```python
from build123d import *

# Parameters (mm, degrees)
BASE_PLATE_AND_PORTS_2_R   = 0.35
BASE_PLATE_AND_PORTS_2_R_2 = 1.075
BASE_PLATE_AND_PORTS_DEPTH = 1.5
BOSS_EXTRUDE1_DEPTH        = 15
RESERVOIRS_3_W             = 0.5
RESERVOIRS_3_H             = 12
BOSS_EXTRUDE2_DEPTH        = 13


with BuildPart() as part:
    # Base-plate and ports 2 → Base plate and ports (new, symmetric)
    with BuildSketch(Plane(origin=(0, 0, 0), x_dir=(1, 0, 0), z_dir=(0, 1, 0))):
        with BuildLine():
            Line((-16, -7), (-16, 7))
            ThreePointArc((-16, 7), (-15.560660172, 8.060660172), (-14.5, 8.5))
            Line((-14.5, 8.5), (-3.175, 8.5))
            ThreePointArc((-3.175, 8.5), (-2.379504871, 8.829504871), (-2.05, 9.625))
            ThreePointArc((-2.05, 9.625), (0, 11.675), (2.05, 9.625))
            ThreePointArc((2.05, 9.625), (2.379504871, 8.829504871), (3.175, 8.5))
            Line((3.175, 8.5), (14.5, 8.5))
            ThreePointArc((14.5, 8.5), (15.560660172, 8.060660172), (16, 7))
            Line((16, 7), (16, -7))
            ThreePointArc((16, -7), (15.560660172, -8.060660172), (14.5, -8.5))
            Line((14.5, -8.5), (12.175, -8.5))
            ThreePointArc((12.175, -8.5), (11.379504871, -8.829504871), (11.05, -9.625))
            ThreePointArc((11.05, -9.625), (9, -11.675), (6.95, -9.625))
            ThreePointArc((6.95, -9.625), (6.620495129, -8.829504871), (5.825, -8.5))
            Line((5.825, -8.5), (-5.825, -8.5))
            ThreePointArc((-5.825, -8.5), (-6.620495129, -8.829504871), (-6.95, -9.625))
            ThreePointArc((-6.95, -9.625), (-9, -11.675), (-11.05, -9.625))
            ThreePointArc((-11.05, -9.625), (-11.379504871, -8.829504871), (-12.175, -8.5))
            Line((-12.175, -8.5), (-14.5, -8.5))
            ThreePointArc((-14.5, -8.5), (-15.560660172, -8.060660172), (-16, -7))
        make_face()
        with Locations(Location((-10.5, 3, 0), (0, 0, 270))):
            Circle(BASE_PLATE_AND_PORTS_2_R, mode=Mode.SUBTRACT)
        with Locations(Location((0, 3, 0), (0, 0, 270))):
            Circle(BASE_PLATE_AND_PORTS_2_R, mode=Mode.SUBTRACT)
        with Locations(Location((10.5, 3, 0), (0, 0, 270))):
            Circle(BASE_PLATE_AND_PORTS_2_R, mode=Mode.SUBTRACT)
        with Locations(Location((0, -3, 0), (0, 0, 270))):
            Circle(BASE_PLATE_AND_PORTS_2_R, mode=Mode.SUBTRACT)
        with Locations(Location((10.5, -3, 0), (0, 0, 270))):
            Circle(BASE_PLATE_AND_PORTS_2_R, mode=Mode.SUBTRACT)
        with Locations(Location((-10.5, -3, 0), (0, 0, 270))):
            Circle(BASE_PLATE_AND_PORTS_2_R, mode=Mode.SUBTRACT)
        with Locations(Location((0, 9.625, 0), (0, 0, 270))):
            Circle(BASE_PLATE_AND_PORTS_2_R_2, mode=Mode.SUBTRACT)
        with Locations(Location((-9, -9.625, 0), (0, 0, 270))):
            Circle(BASE_PLATE_AND_PORTS_2_R_2, mode=Mode.SUBTRACT)
        with Locations(Location((9, -9.625, 0), (0, 0, 270))):
            Circle(BASE_PLATE_AND_PORTS_2_R_2, mode=Mode.SUBTRACT)
    extrude(amount=BASE_PLATE_AND_PORTS_DEPTH, both=True)

    # Reservoirs → Boss-Extrude1 (add)
    with BuildSketch(Plane(origin=(0, 1.5, 0), x_dir=(1, 0, 0), z_dir=(0, 1, 0))):
        with BuildLine():
            Line((-13.5, 6.5), (13.5, 6.5))
            ThreePointArc((13.5, 6.5), (13.853553391, 6.353553391), (14, 6))
            Line((14, 6), (14, -6))
            ThreePointArc((14, -6), (13.853553391, -6.353553391), (13.5, -6.5))
            Line((13.5, -6.5), (-13.5, -6.5))
            ThreePointArc((-13.5, -6.5), (-13.853553391, -6.353553391), (-14, -6))
            Line((-14, -6), (-14, 6))
            ThreePointArc((-14, 6), (-13.853553391, 6.353553391), (-13.5, 6.5))
        make_face()
        Polygon((-4.333333333, -6), (4.333333333, -6), (4.833333333, -6), (13.5, -6), (13.5, 6), (4.833333333, 6), (4.333333333, 6), (-4.333333333, 6), (-4.833333333, 6), (-13.5, 6), (-13.5, -6), (-4.833333333, -6), align=None, mode=Mode.SUBTRACT)
    extrude(amount=BOSS_EXTRUDE1_DEPTH)

    # Reservoirs<3> → Boss-Extrude2 (add)
    with BuildSketch(Plane(origin=(0, 1.5, 0), x_dir=(1, 0, 0), z_dir=(0, 1, 0))):
        with Locations((-4.583333333, 0)):
            Rectangle(RESERVOIRS_3_W, RESERVOIRS_3_H)
        with Locations((4.583333333, 0)):
            Rectangle(RESERVOIRS_3_W, RESERVOIRS_3_H)
    extrude(amount=BOSS_EXTRUDE2_DEPTH)


solid = part.part
```
Work out the finished part from the listing and answer in its coordinate system (mm). A direction names the side the tool comes from. Round coordinates to 2 decimals unless told otherwise and drop trailing zeros. Write each loop counter-clockwise with the first axis right and the second up, starting at its lowest first coordinate (ties: lowest second). Pieces come first, ordered by that corner, then holes.
1) A cutting plane is placed at B-B on z = 3. Give the number of separate pieces and of enclosed holes in the cut face, and give its area (3 significant figures).
2) A cutting plane is placed at D-D on y = 9.25. Determine the outline of the cut face in (x, z), and give its area (3 significant figures).
3) A cutting plane is placed at C-C on x = 9. Determine the outline of the cut face in (y, z) (3 decimals), and give its area (3 significant figures).
4) Consider probe 1 along X at (y, z) = (-0.45, 3); probe 2 along X at (y, z) = (14, -1); probe 3 along Z at (x, y) = (10, 2.5). Determine where each line is inside the solid, lowest interval first.
5) Determine the mould class of faces 5 (the face through (9, 0, -8.5)), 6 (the face through (14, 9, 0)), 7 (the face through (7.95, -0.02, 9.39)) for opening direction Z: pulls with the +Z half, pulls with the -Z half, needs draft (parallel to the pull), parting line crosses it, or undercut.
6) A cutting plane is placed at A-A on x = 0. Determine the outline of the cut face in (y, z) (3 decimals), and give its area (3 significant figures).
7) Flat-ended cylindrical pins translate along their axes: P1, Ø10, axis at x = 1, z = 0, coming from the +Y side; P2, Ø6, axis at x = -9, y = 9, coming from the -Z side; P3, Ø2.5, axis at x = -2, y = 0.5, coming from the +Z side; P4, Ø10, axis at y = 5, z = -4, coming from the -X side. Find the tip coordinate at first contact, or state that the pin passes through.
8) Which of the six approach directions +Z, -Z, +X, -X, +Y, -Y give full straight-line access (tool end or side, diameter ignored) to faces 1 (the face through (-13, 0, 8.5)), 2 (the face through (6.63, 0.02, 8.84)), 3 (the face through (0, 9, -6.5)), 4 (the face through (9, 1.5, 0))?
Entries:
1. separate pieces: 4
1. enclosed holes: 0
1. area: 118 mm2
2. outline: (-14, -6) arc R0.5 ccw to (-13.5, -6.5) - (13.5, -6.5) arc R0.5 ccw to (14, -6) - (14, 6) arc R0.5 ccw to (13.5, 6.5) - (-13.5, 6.5) arc R0.5 ccw to (-14, 6) - close; hole (-13.5, -6) - (-4.83, -6) - (-4.83, 6) - (-13.5, 6) - close; hole (-4.33, -6) - (4.33, -6) - (4.33, 6) - (-4.33, 6) - close; hole (4.83, -6) - (13.5, -6) - (13.5, 6) - (4.83, 6) - close
2. area: 51.8 mm2
3. outline: (-1.5, -8.5) - (1.5, -8.5) - (1.5, -6.5) - (16.5, -6.5) - (16.5, -6) - (1.5, -6) - (1.5, 6) - (16.5, 6) - (16.5, 6.5) - (1.5, 6.5) - (1.5, 8.55) - (-1.5, 8.55) - close; (-1.5, 10.7) - (1.5, 10.7) - (1.5, 11.675) - (-1.5, 11.675) - close
3. area: 69.1 mm2
4. probe 1: x = -16 to -10.85, -10.15 to -0.35, 0.35 to 10.15, 10.85 to 16
4. probe 2: x = -14 to -13.5, -4.83 to -4.33, 4.33 to 4.83, 13.5 to 14
4. probe 3: z = -6.5 to -6, 6 to 6.5
5. face 5: pulls with the -Z half
5. face 6: needs draft
5. face 7: undercut
6. outline: (-1.5, -11.675) - (1.5, -11.675) - (1.5, -10.7) - (-1.5, -10.7) - close; (-1.5, -8.55) - (1.5, -8.55) - (1.5, -6.5) - (16.5, -6.5) - (16.5, -6) - (1.5, -6) - (1.5, -3.35) - (-1.5, -3.35) - close; (-1.5, -2.65) - (1.5, -2.65) - (1.5, 2.65) - (-1.5, 2.65) - close; (-1.5, 3.35) - (1.5, 3.35) - (1.5, 6) - (16.5, 6) - (16.5, 6.5) - (1.5, 6.5) - (1.5, 8.5) - (-1.5, 8.5) - close
6. area: 64.9 mm2
7. P1: stops at y = 14.5
7. P2: stops at z = -6.5
7. P3: stops at z = 8.5
7. P4: stops at x = -16
8. face 1: +Z, -X, +Y, -Y
8. face 2: +Z, +Y, -Y
8. face 3: -Z, +X, -X, +Y
8. face 4: +Y
